from build123d import *

# Parameters (mm, degrees)
ENLEV_MAT_EXTRU_1_DEPTH      = 1
ENLEV_MAT_EXTRU_1_DEPTH_BACK = 10
ESQUISSE3_W                  = 2
ESQUISSE3_H                  = 10
CHANFREIN1_SIZE              = 0.4
ENL_V_MAT_EXTRU_1_DEPTH      = 1


with BuildPart() as part:
    # Esquisse1 → Base-R_volution (revolve)
    with BuildSketch(Plane(origin=(0, 0, 0), x_dir=(1, 0, 0), z_dir=(0, 1, 0)), mode=Mode.PRIVATE) as base_r_volution_sk:
        with BuildLine():
            Line((0, 0), (2, 0))
            Line((2, 0), (3.680261609, 1.680261609))
            ThreePointArc((3.680261609, 1.680261609), (3.699400389, 1.768324283), (3.691522185, 1.858097672))
            ThreePointArc((3.691522185, 1.858097672), (1.958780857, 2.831960417), (0, 3.169567743))
            Line((0, 3.169567743), (0, 0))
        make_face()
    revolve(base_r_volution_sk.sketch.rotate(Axis((0, 0, 0), (0, 0, -1)), 180), axis=Axis((0, 0, 0), (0, 0, -1)))

    # Esquisse2 → Enlev. mat.-Extru.1 (cut, two sides: drawn at the far end of the back side and taken through both)
    with BuildSketch(Plane.XY.offset(-3.1).offset(-ENLEV_MAT_EXTRU_1_DEPTH_BACK)):
        Polygon((0.6, -0.6), (0.6, -2.35), (-0.6, -2.35), (-0.6, -0.6), (-2.35, -0.6), (-2.35, 0.6), (-0.6, 0.6), (-0.6, 2.35), (0.6, 2.35), (0.6, 0.6), (2.35, 0.6), (2.35, -0.6), align=None)
    extrude(amount=ENLEV_MAT_EXTRU_1_DEPTH + ENLEV_MAT_EXTRU_1_DEPTH_BACK, mode=Mode.SUBTRACT)

    # Esquisse3 → Boss.-R_vol.1 (revolve)
    with BuildSketch(Plane(origin=(0, 0, 0), x_dir=(1, 0, 0), z_dir=(0, 1, 0)), mode=Mode.PRIVATE) as boss_r_vol_1_sk:
        with Locations((1, -5)):
            Rectangle(ESQUISSE3_W, ESQUISSE3_H)
    revolve(boss_r_vol_1_sk.sketch.rotate(Axis((0, 0, 0), (0, 0, 1)), 345.677280022), axis=Axis((0, 0, 0), (0, 0, 1)))

    # Chanfrein1
    chanfrein1_edges = [part.edges().sort_by_distance(p)[0] for p in [
        (-1.937835421, 0.494766491, 10),
    ]]
    chamfer(chanfrein1_edges, length=CHANFREIN1_SIZE)

    # Esquisse6 → Enl_v. mat.-Extru.1 (cut)
    with BuildSketch(Plane(origin=(0, 0, -2.1), x_dir=(-1, 0, 0), z_dir=(0, 0, -1))):
        Polygon((2.35, 0.6), (0.6, 0.6), (0.6, 2.35), (-0.6, 2.35), (-0.6, 0.6), (-2.35, 0.6), (-2.35, -0.6), (-0.6, -0.6), (-0.6, -2.35), (0.6, -2.35), (0.6, -0.6), (2.35, -0.6), align=None)
    extrude(amount=-ENL_V_MAT_EXTRU_1_DEPTH, mode=Mode.SUBTRACT)


solid = part.part
Here's how the part is built. I have some questions about the finished solid (model axes, mm). A direction names the side the tool comes from. Coordinates: 2 decimals unless noted, no trailing zeros. Write each loop counter-clockwise with the first axis right and the second up, starting at its lowest first coordinate (ties: lowest second). Pieces come first, ordered by that corner, then holes.
1) I'm going to push flat-ended pins straight in: pin 1 (2 mm diameter, centred on y = 0.5, z = 6.5, fed in from +X); pin 2 (1.9 mm diameter, centred on y = 1.5, z = -2.5, fed in from +X); pin 3 (4 mm diameter, centred on y = 2.5, z = 1.5, fed in from -X). Where does each tip first touch, or does it pass through?
Filled in:
pin 1: stops at x = 2
pin 2: stops at x = 3.6
pin 3: stops at x = -1.94
2) If we section it at C-C (z = 1.25): List the corners of the cut face in (x, y) for me, plus the area to 3 significant figures.
Filled in:
outline: circle Ø4 at (0, 0)
area: 12.6 mm2
3) If I drill on line 1 (Y direction, x = 0.25, z = -1.75); line 2 (Z direction, x = -0.5, y = 1.5); line 3 (Y direction, x = 1.25, z = -1.75), over which ranges is the centre line in solid material (lowest first)?
Filled in:
line 1: y = -3.69 to -2.35, 2.35 to 3.69
line 2: z = -1.1 to 10
line 3: y = -3.48 to -0.6, 0.6 to 3.48
4) Thinking about a two-plate mould opening in X: for faces 3 (the face through (0.46, -2.06, -0.11)), 4 (the face through (2.35, 0, -2)), 5 (the face through (0, 0, 10)), which applies, +X half, -X half, draft (parallel to the pull), parting line (faces both ways), or undercut?
Filled in:
face 3: parting line
face 4: undercut
face 5: draft
5) Which directions (+Z, -Z, +X, -X, +Y, -Y) give clear straight access to the entire face, cutting with the end or side of a thin tool? Please do faces 1 (the face through (0, -2, 5)), 2 (the face through (0, 0, -1.1)).
Filled in:
face 1: +Z
face 2: -Z
6) If we section it at A-A (x = 0): List the corners of the cut face in (y, z) for me, plus the area to 3 significant figures.
Filled in:
outline: (-3.69, -1.86) arc R5.85 ccw to (-2.35, -2.68) - (-2.35, -1.1) - (2.35, -1.1) - (2.35, -2.68) arc R5.85 ccw to (3.69, -1.86) arc R0.3 ccw to (3.68, -1.68) - (2, 0) - (2, 9.6) - (1.6, 10) - (-1.6, 10) - (-2, 9.6) - (-2, 0) - (-3.68, -1.68) arc R0.3 ccw to start
area: 48.3 mm2
